Work out the finished part from the listing and answer in its coordinate system (mm). Coordinates: 2 decimals unless noted, no trailing zeros. Order: outer loops, then holes, each group sorted by start corner. A loop starts at its lowest first (then second) coordinate and runs counter-clockwise, first axis right, second up. Notation, with made-up numbers: (-16, 50.5) -> (31, 50.5) arc R28 ccw to (31, 76.5) -> close; hole circle Ø1 at (77.5, 89). An arc over 180 degrees is marked (long way). Write item = value, one per line. Start each with the question number.
Q1. Straight lines are drawn through the part: L1, parallel to Z at x = 0.5, y = 0; L2, parallel to Y at x = 0.15, z = 3.5; L3, parallel to Y at x = 0.55, z = -2. For each, find the intervals that lie inside material, in ascending order. Write a range as from..to.
Q2. A flat-ended cylindrical pin translates along its axis: pin 1 (6 mm diameter, centred on y = 1, z = -4.5, fed in from -X). Find the tip coordinate at first contact, or state that the pin passes through.
Q3. The part is cut by section A-A, the plane y = 0. Determine the outline of the cut face in (x, z), plus the area to 3 significant figures.
Q4. The part is cut by section C-C, the plane y = 3.75. Determine the outline of the cut face in (x, z).
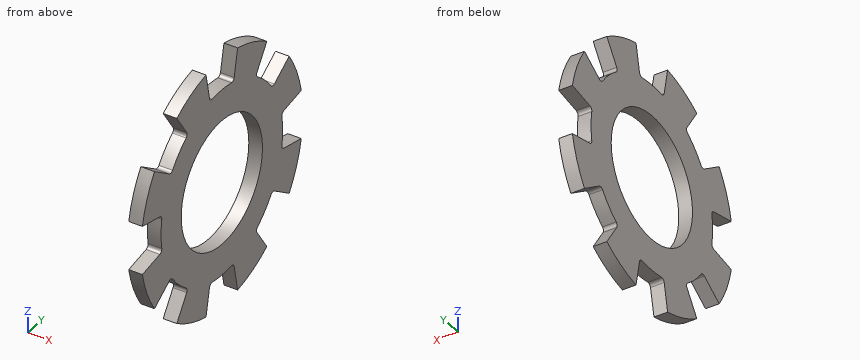
Autodesk Inventor part; units mm, degrees
ref_plane "YZ Plane" through (0, 0, 0) normal (1, 0, 0) x (0, 1, 0)
ref_plane "XZ Plane" through (0, 0, 0) normal (0, 1, 0) x (-1, 0, 0)
ref_plane "XY Plane" through (0, 0, 0) normal (0, 0, 1) x (1, 0, 0)
sketch "Sketch1" plane through (0, 0, 0) normal (1, 0, 0) x (0, 1, 0)
  circle A0 centre (0, 0) radius 6.477
  circle A1 centre (0, 0) radius 3.2512
  dimension "d0" = 12.954
  dimension "d1" = 6.5024
extrude "Body" add sketch "Sketch1" along normal blind 0.7112
sketch "Sketch2" plane through (0.7112, 0, 0) normal (1, 0, 0) x (0, 0, -1)
  circle A0 centre (0, 0) radius 6.477
  line L0 (0, 0) -> (0, 6.477) construction
  arc A1 (1.2636, 6.3525) -> (-1.2636, 6.3525) centre (0, 0) ccw
  arc A2 (0.9489, 4.7706) -> (-0.9489, 4.7706) centre (0, 0) ccw
  line L1 (-0.9489, 4.7706) -> (-1.2636, 6.3525)
  line L2 (0.9489, 4.7706) -> (1.2636, 6.3525)
  line L3 (-0.9489, 4.7706) -> (0, 0) construction
  line L4 (0, 0) -> (0.9489, 4.7706) construction
  dimension "d4" = 22.5
  dimension "d5" = 9.7282
extrude "Cut" cut sketch "Sketch2" against normal through all contours L2 A2 L1 A0 picked at (-0.106, 5.9266)
fillet "Fillet1" radius 0.1943 2 edges at (0.3556, 4.7706, 0.9489) (0.3556, 4.7706, -0.9489)
pattern_circular "Cuts" count 8 over 360 about axis through (0, 0, 0) along (1, 0, 0) of "Cut", "Fillet1"
equation "\"d0\" = SD2"
equation "\"d1\" = SD1"
equation "\"d2\" = SD"
equation "\"d5\" = 0.5 * SD2 + 0.5 * SD1"
equation "\"d6\" = SD"
equation "\"d8\" = 0.015 * SD2"
equation "\"SD\" = 0.7112"
equation "\"SD1\" = 6.5024"
equation "\"SD2\" = 12.954"
equation "\"NND\" = 6.35"
properties part number "ASME B18.21.1 - 1/4. Carbon Steel" material "Steel, Mild"
Model answer:
q1.L1 = -4.86..-3.25, 3.25..4.86
q1.L2 = -5.45..-5.24, -3.38..3.38, 5.24..5.45
q1.L3 = -6.16..-2.56, 2.56..6.16
q2.pin_1 = 0
q3.outline = (0, -4.86) -> (0.71, -4.86) -> (0.71, -3.25) -> (0, -3.25) -> close; (0, 3.25) -> (0.71, 3.25) -> (0.71, 4.86) -> (0, 4.86) -> close
q3.area = 2.29 mm2
q4.outline = (0, -3.1) -> (0.71, -3.1) -> (0.71, 3.1) -> (0, 3.1) -> close
